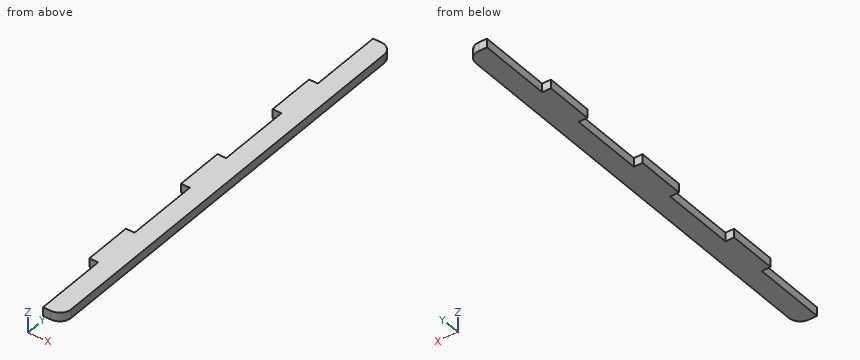
```python
from build123d import *

# Parameters (mm, degrees)
BOSS_EXTRUDE1_DEPTH = 5.35


with BuildPart() as part:
    # Model → Boss-Extrude1 (new body)
    with BuildSketch(Plane.XY):
        with BuildLine():
            Line((10.350000329, 268.999993801), (5.350000225, 268.999993801))
            Line((5.350000225, 268.999993801), (5.350000225, 223.999992013))
            Line((5.350000225, 223.999992013), (0, 223.999992013))
            Line((0, 223.999992013), (0, 194.333329797))
            Line((0, 194.333329797), (5.350000225, 194.333329797))
            Line((5.350000225, 194.333329797), (5.350000225, 149.333328009))
            Line((5.350000225, 149.333328009), (0, 149.333328009))
            Line((0, 149.333328009), (0, 119.666665792))
            Line((0, 119.666665792), (5.350000225, 119.666665792))
            Line((5.350000225, 119.666665792), (5.350000225, 74.666664004))
            Line((5.350000225, 74.666664004), (0, 74.666664004))
            Line((0, 74.666664004), (0, 44.999986887))
            Line((0, 44.999986887), (5.350000225, 44.999986887))
            Line((5.350000225, 44.999986887), (5.350000225, 0))
            Line((5.350000225, 0), (10.350000113, 0))
            ThreePointArc((10.350000113, 0), (15.299747721, 2.050252455), (17.350000329, 7))
            Line((17.350000329, 7), (17.350000329, 261.999993585))
            ThreePointArc((17.350000329, 261.999993585), (15.299747874, 266.949741193), (10.350000329, 268.999993801))
        make_face()
    extrude(amount=BOSS_EXTRUDE1_DEPTH)


solid = part.part
```
Build history of the part. All positions in model axes, mm. Coordinates: 2 decimals unless noted, no trailing zeros. Order: outer loops, then holes, each group sorted by start corner. A loop starts at its lowest first (then second) coordinate and runs counter-clockwise, first axis right, second up.
Item 1: Drop flat-ended pins along their axis: pin 1 Ø2.5 at (x, z) = (3, 3) entering from -Y; pin 2 Ø2.5 at (y, z) = (91.5, 3.5) entering from -X; pin 3 Ø2 at (x, z) = (8.5, 3.5) entering from -Y; pin 4 Ø2.5 at (x, z) = (3.5, 3) entering from +Y. Give the stop position or say it passes through.
Filled in:
pin 1: stops at y = 45
pin 2: stops at x = 5.35
pin 3: stops at y = 0
pin 4: stops at y = 224
Item 2: Saw through at A-A on z = 2.5. List the corners of the cut face in (x, y), then the cut area to 3 significant figures.
Filled in:
outline: (0, 45) - (5.35, 45) - (5.35, 0) - (10.35, 0) arc R7 ccw to (17.35, 7) - (17.35, 262) arc R7 ccw to (10.35, 269) - (5.35, 269) - (5.35, 224) - (0, 224) - (0, 194.33) - (5.35, 194.33) - (5.35, 149.33) - (0, 149.33) - (0, 119.67) - (5.35, 119.67) - (5.35, 74.67) - (0, 74.67) - close
area: 3,680 mm2
Item 3: Drill centre lines: L1, parallel to Y at x = 5.25, z = 1.25; L2, parallel to Y at x = 11, z = 4.25; L3, parallel to X at y = 42, z = 3.4. Where is each one in solid material? Low to high.
Filled in:
L1: y = 45 to 74.67, 119.67 to 149.33, 194.33 to 224
L2: y = 0.03 to 268.97
L3: x = 5.35 to 17.35
Item 4: Saw through at B-B on y = 160. List the corners of the cut face in (x, z), then the cut area to 3 significant figures.
Filled in:
outline: (5.35, 0) - (17.35, 0) - (17.35, 5.35) - (5.35, 5.35) - close
area: 64.2 mm2
